Geometry: final body of the model. Coordinates: model frame, mm. Face numbers are marked on the shaded views. A direction names the side the tool comes from. Round coordinates to 2 decimals unless told otherwise and drop trailing zeros. Write each loop counter-clockwise with the first axis right and the second up, starting at its lowest first coordinate (ties: lowest second). Pieces come first, ordered by that corner, then holes. Notation, with made-up numbers: (30.5, 10.5) -> (89.5, 10.5) arc R20 ccw to (89.5, 19.5) -> close; hole circle Ø11 at (-8, 43). An arc over 180 degrees is marked (long way). One line per item, written item: value. Start each with the question number.
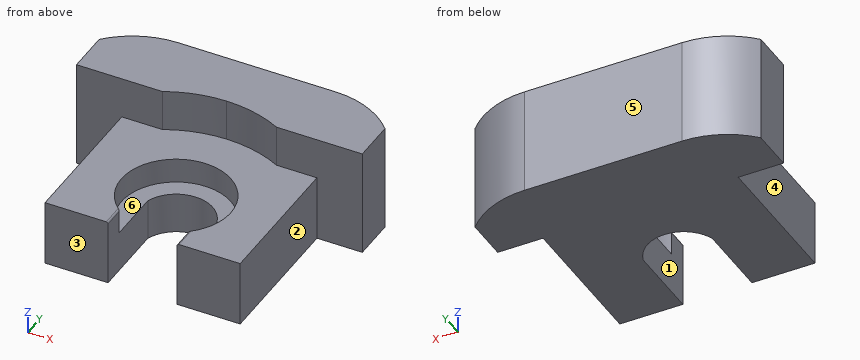
from build123d import *

# Parameters (mm, degrees)
F1_DEPTH = 2.35
F2_DEPTH = 3.78
F3_DEPTH = 6.16
F4_R     = 0.1
F5_R     = 0.1


# Not quite as in the source:
# - a feature names something its author has since deleted; it is built from what else it names


with BuildPart() as f1:
    # F0 (on Top) → F1 (new body)
    with BuildSketch(Plane.XY):
        with BuildLine():
            Line((0.6766474014, -1.6654146139), (0.6766474014, -4.7543960131))
            ThreePointArc((0.6766474014, -4.7543960131), (1.524544849, -3.6730954673), (1.8266474014, -2.3326198054))
            ThreePointArc((1.8266474014, -2.3326198054), (-2.6388282605, 0.4902776422), (-3.2733525986, -4.7543960131))
            Line((-3.2733525986, -4.7543960131), (-3.2733525986, -1.6654146139))
            ThreePointArc((-3.2733525986, -1.6654146139), (-1.2983525986, -0.247964494), (0.6766474014, -1.6654146139))
        make_face()
    extrude(amount=F1_DEPTH)

    # F0 (on Top) → F2 (join)
    with BuildSketch(Plane.XY):
        with BuildLine():
            Line((4.2766474014, -5.9583943095), (4.2766474014, 2.3416056905))
            Line((4.2766474014, 2.3416056905), (1.9666474014, 2.3416056905))
            ThreePointArc((1.9666474014, 2.3416056905), (0.3815359204, 2.9330616855), (-1.2983525986, 3.1339924307))
            ThreePointArc((-1.2983525986, 3.1339924307), (-2.9782411177, 2.9330616855), (-4.5633525986, 2.3416056905))
            Line((-4.5633525986, 2.3416056905), (-6.8733525986, 2.3416056905))
            Line((-6.8733525986, 2.3416056905), (-6.8733525986, -5.9583943095))
            Line((-6.8733525986, -5.9583943095), (-3.2733525986, -5.9583943095))
            Line((-3.2733525986, -5.9583943095), (-3.2733525986, -4.7543960131))
            ThreePointArc((-3.2733525986, -4.7543960131), (-2.6388282605, 0.4902776422), (1.8266474014, -2.3326198054))
            ThreePointArc((1.8266474014, -2.3326198054), (1.524544849, -3.6730954673), (0.6766474014, -4.7543960131))
            Line((0.6766474014, -4.7543960131), (0.6766474014, -5.9583943095))
            Line((0.6766474014, -5.9583943095), (4.2766474014, -5.9583943095))
        make_face()
    extrude(amount=F2_DEPTH)

    # F0 (on Top) → F3 (join)
    with BuildSketch(Plane.XY):
        with BuildLine():
            ThreePointArc((-4.5633525986, 2.3416056905), (-2.9782411177, 2.9330616855), (-1.2983525986, 3.1339924307))
            Line((-1.2983525986, 3.1339924307), (-1.2983525986, 4.7916056905))
            Line((-1.2983525986, 4.7916056905), (-9.4633525986, 4.7916056905))
            Line((-9.4633525986, 4.7916056905), (-9.4633525986, 2.3416056905))
            Line((-9.4633525986, 2.3416056905), (-6.8733525986, 2.3416056905))
            Line((-6.8733525986, 2.3416056905), (-4.5633525986, 2.3416056905))
        make_face()
        with BuildLine():
            Line((1.9666474014, 2.3416056905), (4.2766474014, 2.3416056905))
            Line((4.2766474014, 2.3416056905), (6.8666474014, 2.3416056905))
            Line((6.8666474014, 2.3416056905), (6.8666474014, 4.7916056905))
            Line((6.8666474014, 4.7916056905), (-1.2983525986, 4.7916056905))
            Line((-1.2983525986, 4.7916056905), (-1.2983525986, 3.1339924307))
            ThreePointArc((-1.2983525986, 3.1339924307), (0.3815359204, 2.9330616855), (1.9666474014, 2.3416056905))
        make_face()
        with BuildLine():
            Line((-1.2983525986, 4.7916056905), (6.8666474014, 4.7916056905))
            ThreePointArc((6.8666474014, 4.7916056905), (5.2036474014, 5.9830772848), (3.2016474014, 6.4039924307))
            Line((3.2016474014, 6.4039924307), (-1.2983525986, 6.4039924307))
            Line((-1.2983525986, 6.4039924307), (-1.2983525986, 4.7916056905))
        make_face()
        with BuildLine():
            Line((-9.4633525986, 4.7916056905), (-1.2983525986, 4.7916056905))
            Line((-1.2983525986, 4.7916056905), (-1.2983525986, 6.4039924307))
            Line((-1.2983525986, 6.4039924307), (-5.7983525986, 6.4039924307))
            ThreePointArc((-5.7983525986, 6.4039924307), (-7.8003525986, 5.9830772848), (-9.4633525986, 4.7916056905))
        make_face()
    extrude(amount=F3_DEPTH)

    # F4
    f4_edges = [f1.edges().sort_by_distance(p)[0] for p in [
        (0.676647, -5.356395, 3.78),
    ]]
    fillet(f4_edges, radius=F4_R)

    # F5
    f5_edges = [f1.edges().sort_by_distance(p)[0] for p in [
        (-3.273353, -5.356395, 3.78),
    ]]
    fillet(f5_edges, radius=F5_R)


solid = f1.part
(1) Section query A-A (z = 5.25). Output: boundary loops of the cut face in (x, y), and give its area (3 significant figures).
(2) Line query: probe 1 along Y at (x, z) = (2, 5.5); probe 2 along Z at (x, y) = (4, 0.5); probe 3 along X at (y, z) = (1.5, 1.5). Output: solid intervals per line, ascending.
(3) Pull-direction query (X, two-part tool) for the marked faces 4, 5 and 6; classes: pulls with the +X half, pulls with the -X half, needs draft (parallel to the pull), parting line crosses it, or undercut.
(4) Section query B-B (x = -5). Output: boundary loops of the cut face in (y, z).
(5) Pin query (flat end, axial travel): pin 1 (1.1 mm diameter, centred on y = -2, z = 2, fed in from -X); pin 2 (1.7 mm diameter, centred on x = -2, y = -1, fed in from +Z); pin 3 (1.1 mm diameter, centred on y = -3.5, z = 2, fed in from +X). Return the tip coordinate at first contact, or that it passes through.
(6) Section query D-D (y = -2). Output: boundary loops of the cut face in (x, z), and give its area (3 significant figures).
(7) Section query C-C (y = 0.5). Output: boundary loops of the cut face in (x, z).
(8) Set-up query: the marked faces 1, 2 and 3. Return all of +Z, -Z, +X, -X, +Y, -Y with unobstructed straight access to the full face (end or side cutting, diameter ignored); none if empty.
Results list:
1. outline: (-9.46, 2.34) -> (-4.56, 2.34) arc R7.12 cw to (1.97, 2.34) -> (6.87, 2.34) -> (6.87, 4.79) arc R4.97 ccw to (3.2, 6.4) -> (-5.8, 6.4) arc R4.97 ccw to (-9.46, 4.79) -> close
1. area: 59.2 mm^2
2. probe 1: y = 2.34 to 6.4
2. probe 2: z = 0 to 3.78
2. probe 3: x = -6.87 to 4.28
3. face 4: pulls with the -X half
3. face 5: needs draft
3. face 6: undercut
4. outline: (-5.96, 0) -> (6.4, 0) -> (6.4, 6.16) -> (2.34, 6.16) -> (2.34, 3.78) -> (-5.96, 3.78) -> close
5. pin 1: stops at x = -6.87
5. pin 2: stops at z = 2.35
5. pin 3: stops at x = 4.28
6. outline: (-6.87, 0) -> (-3.27, 0) -> (-3.27, 2.35) -> (-4.41, 2.35) -> (-4.41, 3.78) -> (-6.87, 3.78) -> close; (0.68, 0) -> (4.28, 0) -> (4.28, 3.78) -> (1.81, 3.78) -> (1.81, 2.35) -> (0.68, 2.35) -> close
6. area: 24.0 mm^2
7. outline: (-6.87, 0) -> (4.28, 0) -> (4.28, 3.78) -> (0.02, 3.78) -> (0.02, 2.35) -> (-2.62, 2.35) -> (-2.62, 3.78) -> (-6.87, 3.78) -> close
8. face 1: +Z, -Z, -Y
8. face 2: +Z, -Z, +X, -Y
8. face 3: +Z, -Z, +X, -X, -Y
